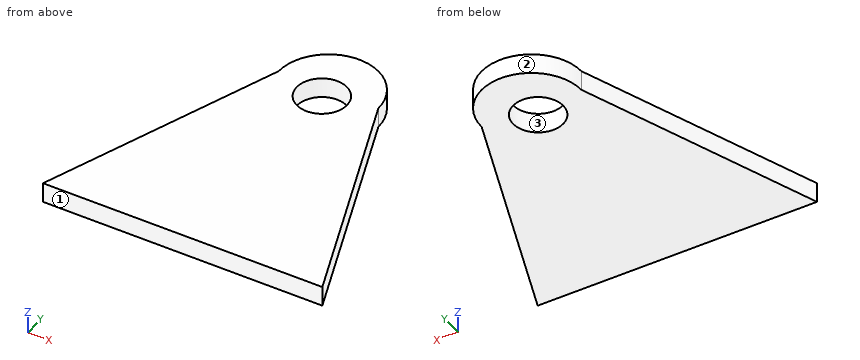
```python
from build123d import *

# Parameters (mm, degrees)
SKETCH1_R           = 50
BOSS_EXTRUDE2_DEPTH = 20
SKETCH2_R           = 25
CUT_EXTRUDE1_DEPTH  = 20


with BuildPart() as part:
    # Sketch1 → Boss-Extrude2 (new body)
    with BuildSketch(Plane.XY):
        with BuildLine():
            Line((88.917270049, 240), (0, 0))
            Line((0, 0), (280, 0))
            Line((280, 0), (188.917270049, 240))
            ThreePointArc((188.917270049, 240), (138.917270049, 190), (88.917270049, 240))
        make_face()
        with Locations((138.917270049, 240)):
            Circle(SKETCH1_R)
    extrude(amount=BOSS_EXTRUDE2_DEPTH)

    # Sketch2 → Cut-Extrude1 (cut)
    with BuildSketch(Plane.XY.offset(20)):
        with Locations((138.81476789, 229.349018501)):
            Circle(SKETCH2_R)
    extrude(amount=-CUT_EXTRUDE1_DEPTH, mode=Mode.SUBTRACT)


solid = part.part
```
CAD build for the part. Positions are in the model's coordinates, mm. Face numbers are marked on the shaded views. Coordinates: 2 decimals unless noted, no trailing zeros. Order: outer loops, then holes, each group sorted by start corner. A loop starts at its lowest first (then second) coordinate and runs counter-clockwise, first axis right, second up.
(1) Saw through at D-D, the plane y = 66.5. Write the cut outline in (x, z).
Solution:
outline: (24.64, 0) - (254.76, 0) - (254.76, 20) - (24.64, 20) - close
(2) Saw through at A-A, the plane y = 235.5. Write the cut outline in (x, z).
Solution:
outline: (87.25, 0) - (114.58, 0) - (114.58, 20) - (87.25, 20) - close; (163.05, 0) - (190.63, 0) - (190.63, 20) - (163.05, 20) - close
(3) Pin check, flat tips, straight feed: pin 1 Ø3 at (x, z) = (133.5, 8.5) entering from +Y; pin 2 Ø2 at (y, z) = (196, 12.5) entering from +X; pin 3 Ø5 at (y, z) = (173.5, 3) entering from -X. Stop position of each tip, or through.
Solution:
pin 1: stops at y = 289.85
pin 2: stops at x = 206
pin 3: stops at x = 63.35
(4) Drill centre lines: L1, parallel to Y at x = 140, z = 14; L2, parallel to X at y = 246, z = 12; L3, parallel to X at y = 219.5, z = 3. Where is each one in solid material? Low to high.
Solution:
L1: y = 0 to 204.38, 254.32 to 289.99
L2: x = 89.28 to 120.17, 157.46 to 188.56
L3: x = 81.32 to 115.84, 161.79 to 196.7
(5) Saw through at C-C, the plane z = 17. Write the cut outline in (x, y).
Solution:
outline: (0, 0) - (280, 0) - (188.92, 240) arc R50 ccw to (88.92, 240) - close; hole circle Ø50 at (138.81, 229.35)
(6) Mould opens along X. For the marked faces 1, 2 and 3 say: released by +X, released by -X, zero draft, split by the parting line, or undercut.
Solution:
face 1: zero draft
face 2: split by the parting line
face 3: undercut
(7) Saw through at B-B, the plane x = 134.5. Write the cut outline in (y, z), and give its area (3 significant figures).
Solution:
outline: (0, 0) - (204.72, 0) - (204.72, 20) - (0, 20) - close; (253.97, 0) - (289.8, 0) - (289.8, 20) - (253.97, 20) - close
area: 4,810 mm2
